The listing builds one solid part. Answer for the finished solid, in the listing's coordinates (mm). A direction names the side the tool comes from. Round coordinates to 2 decimals unless told otherwise and drop trailing zeros. Order: outer loops, then holes, each group sorted by start corner. A loop starts at its lowest first (then second) coordinate and runs counter-clockwise, first axis right, second up. Notation, with made-up numbers: (87, -18.5) -> (110, -18.5) arc R28 ccw to (110, 19.5) -> close; hole circle Ø3 at (74.5, -28.5). An arc over 180 degrees is marked (long way). Answer in a Markdown table with one row per item. Add a question column.
```python
from build123d import *

# Parameters (mm, degrees)
SKETCH1_R           = 50
SKETCH1_R_2         = 30
BOSS_EXTRUDE1_DEPTH = 47


with BuildPart() as part:
    # Sketch1 → Boss-Extrude1 (new body)
    with BuildSketch(Plane.XY):
        with BuildLine():
            Line((-46.727102691, 252.119188355), (-46.727102691, 258.937140002))
            add(Edge.make_bspline(
                [(-22.082294652, 230.189836254), (-33.358154649, 247.131709382), (-46.727102689, 258.937140004)],
                knots=[0, 0, 0, 0.202133658, 0.202133658, 0.202133658], degree=2))
            add(Edge.make_bspline(
                [(-4.870036741, 49.762262229), (-4.393775013, 55.181886992), (-3.493820314, 66.662022051), (-2.529366378, 83.59139057), (-1.982320476, 100.516724073), (-1.858789362, 121.992140621), (-2.814978943, 146.760764163), (-5.156886221, 168.679611703), (-7.775671314, 184.458623381), (-10.08390129, 195.406366158), (-12.704291898, 205.462363583), (-15.117675621, 213.09980662), (-17.165967371, 218.768249548), (-18.756253721, 222.802063426), (-20.120456476, 225.981036836), (-21.236527654, 228.424580455), (-21.795733048, 229.59981685), (-22.082294652, 230.189836254)],
                knots=[0.06256779, 0.06256779, 0.06256779, 0.06256779, 0.087876155, 0.117168207, 0.146460259, 0.17575231, 0.234336414, 0.292920517, 0.322212569, 0.35150462, 0.380796672, 0.410088724, 0.42473475, 0.439380776, 0.454026801, 0.461349814, 0.468672827, 0.468672827, 0.468672827, 0.468672827], degree=3))
            ThreePointArc((-4.870036741, 49.762262229), (33.589419189, 37.037155918), (50, 0))
            add(Edge.make_bspline(
                [(50, 0), (87.107306859, 283.791217757), (-46.727102691, 327.431264092)],
                knots=[0, 0, 0, 0.770439733, 0.770439733, 0.770439733], degree=2))
            Line((-46.727102691, 327.431264091), (-46.727102691, 352.119188355))
            Line((-46.727102691, 352.119188355), (-83.272897309, 352.119188355))
            Line((-83.272897309, 352.119188355), (-83.272897309, 252.119188355))
            Line((-83.272897309, 252.119188355), (-46.727102691, 252.119188355))
        make_face()
        Circle(SKETCH1_R)
        Circle(SKETCH1_R_2, mode=Mode.SUBTRACT)
    extrude(amount=BOSS_EXTRUDE1_DEPTH)


solid = part.part
```
Item 1: Find the intervals of material crossed by probe 1 along Y at (x, z) = (-20.5, 32.5); probe 2 along Y at (x, z) = (-26, 38); probe 3 along Y at (x, z) = (0, 26), in increasing order. Write a range as [from, to].
Item 2: The part is cut by section A-A, the plane x = -71. Give the vertices of the cut face in (y, z).
Item 3: Flat-ended cylindrical pins translate along their axes: P1, Ø2, axis at x = -6.5, z = 27.5, coming from the +Y side; P2, Ø10, axis at x = -25.5, z = 25.5, coming from the -Y side; P3, Ø11, axis at x = -63.5, z = 14.5, coming from the -Y side. Find the tip coordinate at first contact, or state that the pin passes through.
Item 4: For a pull along Y with two mould halves and no side action, classify faces 1 (the face through (-46.727, 255, 23)), 2 (the face through (-65, 352.119, 23)), 3 (the face through (-83.273, 303, 23)) as released by +Y, released by -Y, zero draft, split by the parting line, or undercut.
Item 5: A tool of negligible diameter and unlimited length cuts with its end or side. For faces 4 (the face through (-46.727, 340, 23)), 5 (the face through (-29.97, 1.32, 23.17)), from which of +Z, -Z, +X, -X, +Y, -Y can it reach the whole face along a straight path? Write none if from no direction.
Resolved:
| question | item | result |
|---|---|---|
| 1 | probe 1 | [-45.6, -21.9], [21.9, 45.6], [226.8, 315.62] |
| 1 | probe 2 | [-42.71, -14.97], [14.97, 42.71], [235.83, 318.7] |
| 1 | probe 3 | [-50, -30], [30, 300.34] |
| 2 | outline | (252.12, 0) -> (352.12, 0) -> (352.12, 47) -> (252.12, 47) -> close |
| 3 | P1 | y = 306.72 |
| 3 | P2 | y = -45.6 |
| 3 | P3 | y = 252.12 |
| 4 | face 1 | undercut |
| 4 | face 2 | released by +Y |
| 4 | face 3 | zero draft |
| 5 | face 4 | +Z, -Z, +X, +Y |
| 5 | face 5 | +Z, -Z |
